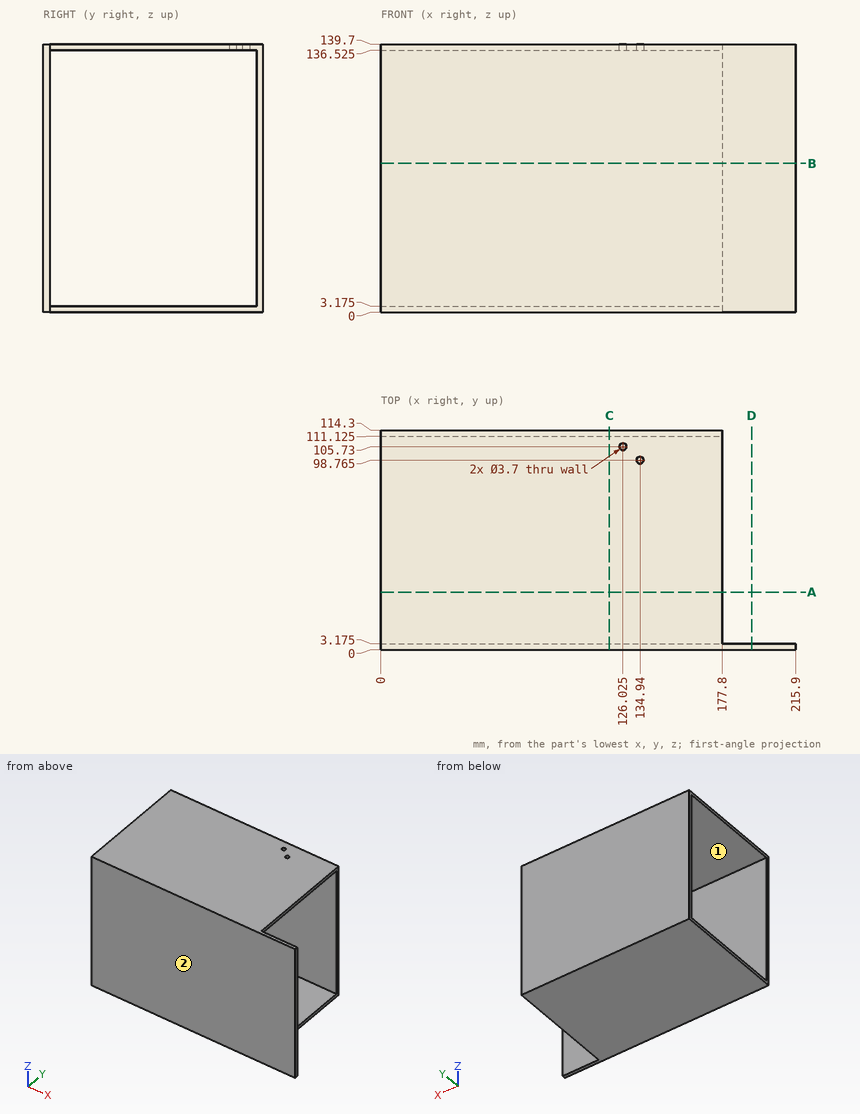
Answer from the drawing. Dimensions are ordinates in mm from the lowest x, y and z of the part. A direction names the side the tool comes from. Round coordinates to 2 decimals unless told otherwise and drop trailing zeros. Order: outer loops, then holes, each group sorted by start corner. A loop starts at its lowest first (then second) coordinate and runs counter-clockwise, first axis right, second up. Notation, with made-up numbers: (-7, -27) -> (10, -27) arc R22 cw to (10, -1) -> close; hole circle Ø4 at (-37, 51.25). An arc over 180 degrees is marked (long way). Answer as CSV lines item,"result".
Q1. Given pin 1 (3 mm diameter, centred on x = 126.02, y = 105.73, fed in from +Z) (3 decimals), flat-ended and moving along its own axis, determine where the tip first touches the part or whether it passes through.
Computed values:
pin 1,"stops at z = 3.175"
Q2. A cutting plane is placed at A-A on y = 30. Determine the outline of the cut face in (x, z) (1 decimal).
Computed values:
outline,"(0, 0) -> (177.8, 0) -> (177.8, 3.2) -> (0, 3.2) -> close; (0, 136.5) -> (177.8, 136.5) -> (177.8, 139.7) -> (0, 139.7) -> close"
Q3. Which of the six approach directions +Z, -Z, +X, -X, +Y, -Y give full straight-line access (tool end or side, diameter ignored) to the marked faces 1 and 2?
Computed values:
face 1,"+X, -X"
face 2,"+Z, -Z, +X, -X, -Y"
Q4. Consider line 1 (Y direction, x = 95, z = 89) (1 decimal); line 2 (Z direction, x = 84, y = 5.5) (1 decimal); line 3 (Y direction, x = 185, z = 15.5) (1 decimal). Determine where each line is inside the solid, lowest interval first. Write a range as from..to.
Computed values:
line 1,"y = 0..3.2, 111.1..114.3"
line 2,"z = 0..3.2, 136.5..139.7"
line 3,"y = 0..3.2"
Q5. A cutting plane is placed at C-C on x = 119. Determine the outline of the cut face in (y, z) (1 decimal), plus the area to 3 significant figures.
Computed values:
outline,"(0, 0) -> (114.3, 0) -> (114.3, 139.7) -> (0, 139.7) -> close; hole (3.2, 3.2) -> (111.1, 3.2) -> (111.1, 136.5) -> (3.2, 136.5) -> close"
area,"1,570 mm^2"
Q6. A cutting plane is placed at B-B on z = 77.5. Determine the outline of the cut face in (x, y) (1 decimal).
Computed values:
outline,"(0, 0) -> (215.9, 0) -> (215.9, 3.2) -> (0, 3.2) -> close; (0, 111.1) -> (177.8, 111.1) -> (177.8, 114.3) -> (0, 114.3) -> close"
Q7. A cutting plane is placed at D-D on x = 193. Determine the outline of the cut face in (y, z) (1 decimal).
Computed values:
outline,"(0, 0) -> (3.2, 0) -> (3.2, 139.7) -> (0, 139.7) -> close"
